Part print with two shaded views. Sizes in mm from the minimum x, y, z corner. A direction names the side the tool comes from. Coordinates: 2 decimals unless noted, no trailing zeros. Order: outer loops, then holes, each group sorted by start corner. A loop starts at its lowest first (then second) coordinate and runs counter-clockwise, first axis right, second up. Notation, with made-up numbers: (5, -6.75) - (40, -6.75) arc R18 cw to (40, 8.25) - close; hole circle Ø2 at (85.25, -29.75). An arc over 180 degrees is marked (long way). Return JSON: item names as keys, results as strings.
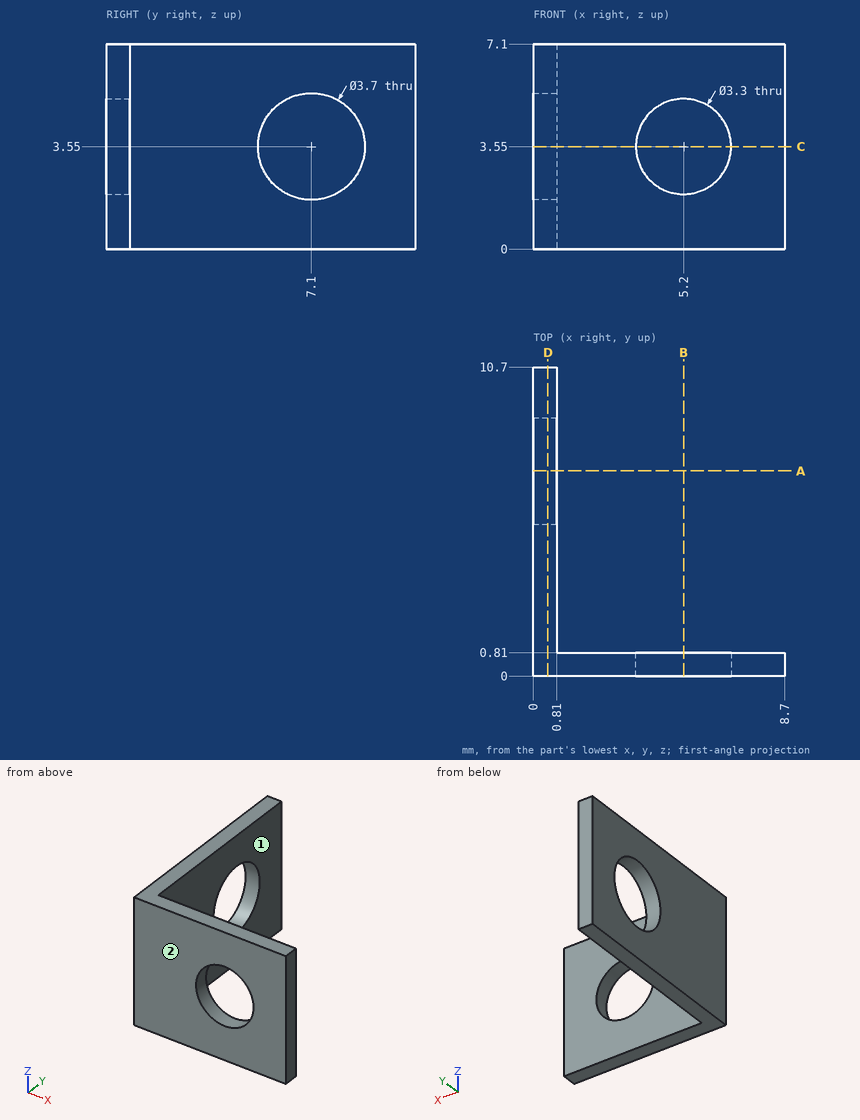
Item 1: Drop a flat-ended pin along its axis: P1, Ø3.5, axis at x = 6.5, z = 5, coming from the +Y side. Give the stop position or say it passes through.
Findings below:
{"P1": "stops at y = 0.81"}
Item 2: Band-saw the part on C-C, the plane z = 3.55. List the corners of the cut face in (x, y).
Findings below:
{"outline": "(0, 0) - (3.55, 0) - (3.55, 0.81) - (0.81, 0.81) - (0.81, 5.25) - (0, 5.25) - close; (0, 8.95) - (0.81, 8.95) - (0.81, 10.7) - (0, 10.7) - close; (6.85, 0) - (8.7, 0) - (8.7, 0.81) - (6.85, 0.81) - close"}
Item 3: Band-saw the part on D-D, the plane x = 0.5. List the corners of the cut face in (y, z), then the cut area to 3 significant figures.
Findings below:
{"outline": "(0, 0) - (10.7, 0) - (10.7, 7.1) - (0, 7.1) - close; hole circle Ø3.7 at (7.1, 3.55)", "area": "65.2 mm²"}
Item 4: Band-saw the part on B-B, the plane x = 5.2. List the corners of the cut face in (y, z).
Findings below:
{"outline": "(0, 0) - (0.81, 0) - (0.81, 1.9) - (0, 1.9) - close; (0, 5.2) - (0.81, 5.2) - (0.81, 7.1) - (0, 7.1) - close"}
Item 5: Band-saw the part on A-A, the plane y = 7.1. List the corners of the cut face in (x, z), then the cut area to 3 significant figures.
Findings below:
{"outline": "(0, 0) - (0.81, 0) - (0.81, 1.7) - (0, 1.7) - close; (0, 5.4) - (0.81, 5.4) - (0.81, 7.1) - (0, 7.1) - close", "area": "2.75 mm²"}
Item 6: Wall check: L1, parallel to Z at x = 5.2, y = 0.65; L2, parallel to Z at x = 0.65, y = 7.1; L3, parallel to Y at x = 0.2, z = 3.55. Give the ranges that are in metal, low to high. Write a range as [from, to].
Findings below:
{"L1": "z = [0, 1.9], [5.2, 7.1]", "L2": "z = [0, 1.7], [5.4, 7.1]", "L3": "y = [0, 5.25], [8.95, 10.7]"}
Item 7: Which spindle directions (+Z, -Z, +X, -X, +Y, -Y) get a long thin tool onto all of the face, cutting with end or side? Do the marked faces 1 and 2. Say none if no direction does.
Findings below:
{"face 1": "+Z, -Z, +X, +Y", "face 2": "+Z, -Z, +X, -X, -Y"}
